Can you work these out from the model? Positions are in its coordinate system, mm. A direction names the side the tool comes from. Coordinates: 2 decimals unless noted, no trailing zeros. Loops run counter-clockwise (first coordinate to the right, second up) from the corner with the lowest first, then second, coordinate; pieces in that order, holes last.
Autodesk Inventor part; units mm, degrees
ref_plane "YZ Plane" through (0, 0, 0) normal (1, 0, 0) x (0, 1, 0)
ref_plane "XZ Plane" through (0, 0, 0) normal (0, 1, 0) x (-1, 0, 0)
ref_plane "XY Plane" through (0, 0, 0) normal (0, 0, 1) x (1, 0, 0)
sketch "Sketch1" plane through (0, 0, 0) normal (0, 1, 0) x (-1, 0, 0)
  line L0 (0, 0) -> (21.3844, -51.6264)
  line L1 (21.3844, -51.6264) -> (47.9015, -40.6426)
  line L2 (47.9015, -40.6426) -> (31.0668, 0)
  line L3 (31.0668, 0) -> (47.9015, 40.6426)
  line L4 (47.9015, 40.6426) -> (21.3844, 51.6264)
  line L5 (21.3844, 51.6264) -> (0, 0)
  line L6 (31.0668, 0) -> (0, 0) construction
  line L7 (17.3204, 0) -> (56.2011, 93.8662) construction
  circle A0 centre (50.7089, 80.6068) radius 3.175
  circle A1 centre (40.9887, 57.1403) radius 3.175
  circle A2 centre (31.2686, 33.6737) radius 3.175
  circle A3 centre (21.5484, 10.2072) radius 3.175
  line L8 (13.0041, 3.7198) -> (13.0041, -3.7198) construction
  line L9 (13.0041, 0) -> (1.9044, 4.5976) construction
  line L10 (32.6076, 3.7198) -> (1.5408, 3.7198) construction
  line L11 (1.5408, -3.7198) -> (32.6076, -3.7198) construction
  circle A4 centre (21.5484, -10.2072) radius 3.175
  circle A5 centre (31.2686, -33.6737) radius 3.175
  dimension "d0" = 28.702
  dimension "d1" = 135
  dimension "d2" = 55.88
  dimension "d3" = 101.6
  dimension "d4" = 6.35
  dimension "d7" = 25.4
  dimension "d12" = 3.7198
  dimension "d13" = 12.7
  dimension "d14" = 12.0142
  dimension "d15" = 12.7
extrude "Plate1" add sketch "Sketch1" along normal blind 3.048 contours L5 L4 L3 L2 L1 L0
fillet "Corner Round1" radius 6.35 1 edges at (0, 1.524, 0)
equation "\"d3\" = 0.5 * CornerLength"
equation "\"BendRadius\" = Thickness"
equation "\"BendReliefWidth\" = Thickness"
equation "\"BendReliefDepth\" = 0.5 * Thickness"
equation "\"CornerReliefSize\" = 4 * Thickness"
equation "\"MinimumRemnant\" = 2 * Thickness"
equation "\"TransitionRadius\" = BendRadius"
equation "\"JacobiRadiusSize\" = BendRadius"
equation "\"GapSize\" = Thickness"
equation "\"d16\" = BendRadius"
properties part number "CornerBracketSheetMetal"
Item 1: Suppose I cut it at D-D, the plane x = -15.5. Please give me the cut outline in (y, z).
Results are:
outline: (0, -37.42) - (3.05, -37.42) - (3.05, 37.42) - (0, 37.42) - close
Item 2: I need wall thicknesses on line 1 along Z through (x, y) = (-23, 1.5); line 2 along X through (y, z) = (2.2, -36.5); line 3 along Z through (x, y) = (-35.5, 1.35). Which ranges of each line are inside material? Lowest first, please.
Results are:
line 1: z = -50.96 to -13.03, -7.38 to 7.38, 13.03 to 50.96
line 2: x = -46.19 to -32.72, -29.82 to -15.12
line 3: z = -45.78 to -10.7, 10.7 to 45.78
Item 3: Suppose I cut it at A-A, the plane z = 35. Please give me the cut outline in (x, y).
Results are:
outline: (-45.56, 0) - (-34.15, 0) - (-34.15, 3.05) - (-45.56, 3.05) - close; (-28.38, 0) - (-14.5, 0) - (-14.5, 3.05) - (-28.38, 3.05) - close
Item 4: We'd pull the mould along X, two halves only. Please class faces 1 (the face through (-24, 0, 1)), 2 (the face through (-30.58, 1.503, -30.574)), 3 (the face through (-0.523, 1.545, 0.035)): +X half, -X half, draft (parallel to the pull), parting line (faces both ways), or undercut.
Results are:
face 1: draft
face 2: undercut
face 3: +X half
Item 5: Suppose I cut it at C-C, the plane y = 0.7. Count the separate pieces of the cut face and the enclosed holes in it, plus the area to 3 significant figures.
Results are:
separate pieces: 1
enclosed holes: 4
area: 2,740 mm2
Item 6: On a 3-axis mill with a long thin cutter (end or side, diameter ignored), from which of +Z, -Z, +X, -X, +Y, -Y can I reach the whole of each face in a straight line? I mean faces 4 (the face through (-39.366, 1.503, 20.037)), 5 (the face through (-11.338, 1.503, 27.373)). Say none if no direction works.
Results are:
face 4: -X, +Y, -Y
face 5: +Z, +X, +Y, -Y
Item 7: Suppose I cut it at B-B, the plane x = -42. Please give me the cut outline in (y, z).
Results are:
outline: (0, -43.09) - (3.05, -43.09) - (3.05, -26.4) - (0, -26.4) - close; (0, 26.4) - (3.05, 26.4) - (3.05, 43.09) - (0, 43.09) - close
